Geometry: final body of the model. Coordinates: model frame, mm. Face numbers are marked on the shaded views. Round coordinates to 2 decimals unless told otherwise and drop trailing zeros. Write each loop counter-clockwise with the first axis right and the second up, starting at its lowest first coordinate (ties: lowest second). Pieces come first, ordered by that corner, then holes. Notation, with made-up numbers: M 46.25,57 L 71.25,57 A13 cw 71.25,67 Z; hole C -13,40.25 d10. An arc over 180 degrees is marked long. Use one line per item in the form item = value. Start each with the question number.
Item 1: Ray query, probe 1 along X at (y, z) = (3.8, 20); probe 2 along Z at (x, y) = (-13.5, -6.25); probe 3 along X at (y, z) = (-5.25, -16.5). Return the intervals inside material, ascending.
Item 2: Section query A-A (y = -10.5). Return loops of the section in (x, z).
Item 3: Section query D-D (y = -2.25). State how many separate pieces and enclosed holes the cut face has, and give its area (3 significant figures).
Item 4: Pin query (flat end, axial travel): pin 1 Ø5 at (y, z) = (-8, 22.5) entering from -X; pin 2 Ø1.3 at (x, z) = (-32.5, -20) entering from +Y; pin 3 Ø0.5 at (x, y) = (-37.5, -5.5) entering from -Z; pin 4 Ø4.5 at (x, z) = (-34.5, 20) entering from -Y. Return the tip coordinate at first contact, or that it passes through.
Item 5: Pull-direction query (Z, two-part tool) for the marked faces 1, 2, 3 and 4; classes: pulls with the +Z half, pulls with the -Z half, needs draft (parallel to the pull), parting line crosses it, or undercut.
Item 6: Section query C-C (x = -13.5). Return loops of the section in (y, z), and give its area (3 significant figures).
Item 7: Section query B-B (z = 1). Return loops of the section in (x, y), and give its area (3 significant figures).
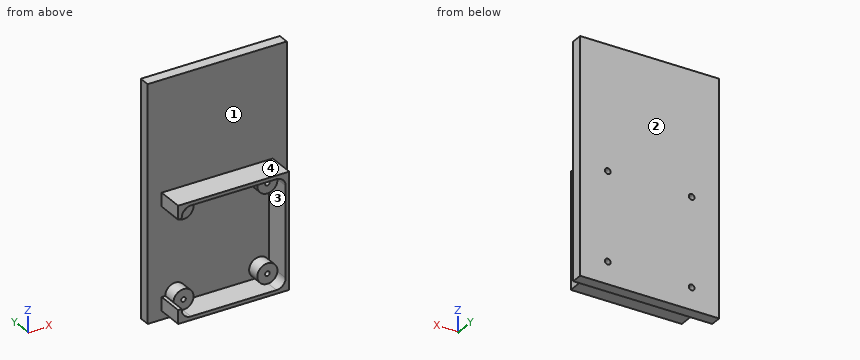
from build123d import *

# Parameters (mm, degrees)
SKETCH3_W           = 63
SKETCH3_H           = 60
BOSS_EXTRUDE3_DEPTH = 5
CUT_EXTRUDE1_REACH  = 56.314
SKETCH4_R           = 1.3
SKETCH9_R           = 4.55
SKETCH9_R_2         = 1.05
BOSS_EXTRUDE5_DEPTH = 6
SKETCH11_W          = 63
SKETCH11_H          = 5
BOSS_EXTRUDE7_DEPTH = 46
SKETCH12_W          = 50.3
SKETCH12_H          = 52.3
BOSS_EXTRUDE8_DEPTH = 12
SKETCH13_W          = 40
SKETCH13_H          = 12
CUT_EXTRUDE4_DEPTH  = 1.62


with BuildPart() as part:
    # Sketch3 → Boss-Extrude3 (new body)
    with BuildSketch(Plane(origin=(0, 0, 0), x_dir=(1, 0, 0), z_dir=(0, 1, 0))):
        with Locations((-13.5, 0)):
            Rectangle(SKETCH3_W, SKETCH3_H)
    extrude(amount=BOSS_EXTRUDE3_DEPTH)

    # Sketch4 → Cut-Extrude1 (cut, up to next)
    with BuildSketch(Plane(origin=(0, 5, 0), x_dir=(1, 0, 0), z_dir=(0, 1, 0)), mode=Mode.PRIVATE) as cut_extrude1_sk1:
        with Locations(Location((-32.5, 20, 0), (0, 0, 270))):
            Circle(SKETCH4_R)
    cut_extrude1_tool1 = extrude(cut_extrude1_sk1.sketch, amount=-CUT_EXTRUDE1_REACH, mode=Mode.PRIVATE) & part.part
    # Sketch4 → Cut-Extrude1 (cut, up to next)
    with BuildSketch(Plane(origin=(0, 5, 0), x_dir=(1, 0, 0), z_dir=(0, 1, 0)), mode=Mode.PRIVATE) as cut_extrude1_sk2:
        with Locations(Location((5.5, 20, 0), (0, 0, 270))):
            Circle(SKETCH4_R)
    cut_extrude1_tool2 = extrude(cut_extrude1_sk2.sketch, amount=-CUT_EXTRUDE1_REACH, mode=Mode.PRIVATE) & part.part
    # Sketch4 → Cut-Extrude1 (cut, up to next)
    with BuildSketch(Plane(origin=(0, 5, 0), x_dir=(1, 0, 0), z_dir=(0, 1, 0)), mode=Mode.PRIVATE) as cut_extrude1_sk3:
        with Locations(Location((5.5, -20, 0), (0, 0, 270))):
            Circle(SKETCH4_R)
    cut_extrude1_tool3 = extrude(cut_extrude1_sk3.sketch, amount=-CUT_EXTRUDE1_REACH, mode=Mode.PRIVATE) & part.part
    # Sketch4 → Cut-Extrude1 (cut, up to next)
    with BuildSketch(Plane(origin=(0, 5, 0), x_dir=(1, 0, 0), z_dir=(0, 1, 0)), mode=Mode.PRIVATE) as cut_extrude1_sk4:
        with Locations(Location((-32.5, -20, 0), (0, 0, 270))):
            Circle(SKETCH4_R)
    cut_extrude1_tool4 = extrude(cut_extrude1_sk4.sketch, amount=-CUT_EXTRUDE1_REACH, mode=Mode.PRIVATE) & part.part
    add(cut_extrude1_tool1.solids().sort_by_distance((-32.5, 5, -20))[0], mode=Mode.SUBTRACT)
    add(cut_extrude1_tool2.solids().sort_by_distance((5.5, 5, -20))[0], mode=Mode.SUBTRACT)
    add(cut_extrude1_tool3.solids().sort_by_distance((5.5, 5, 20))[0], mode=Mode.SUBTRACT)
    add(cut_extrude1_tool4.solids().sort_by_distance((-32.5, 5, 20))[0], mode=Mode.SUBTRACT)

    # Sketch9 → Boss-Extrude5 (add)
    # profile 1 of 4: a face of its own
    with BuildSketch(Plane.XZ):
        with Locations(Location((-32.5, 20, 0), (0, 0, 270))):
            Circle(SKETCH9_R)
        with Locations(Location((-32.5, 20, 0), (0, 0, 270))):
            Circle(SKETCH9_R_2, mode=Mode.SUBTRACT)
    # profile 2 of 4: a face of its own
    with BuildSketch(Plane.XZ):
        with Locations(Location((-32.5, -20, 0), (0, 0, 270))):
            Circle(SKETCH9_R)
        with Locations(Location((-32.5, -20, 0), (0, 0, 270))):
            Circle(SKETCH9_R_2, mode=Mode.SUBTRACT)
    # profile 3 of 4: a face of its own
    with BuildSketch(Plane.XZ):
        with Locations(Location((5.5, 20, 0), (0, 0, 270))):
            Circle(SKETCH9_R)
        with Locations(Location((5.5, 20, 0), (0, 0, 270))):
            Circle(SKETCH9_R_2, mode=Mode.SUBTRACT)
    # profile 4 of 4: a face of its own
    with BuildSketch(Plane.XZ):
        with Locations(Location((5.5, -20, 0), (0, 0, 270))):
            Circle(SKETCH9_R)
        with Locations(Location((5.5, -20, 0), (0, 0, 270))):
            Circle(SKETCH9_R_2, mode=Mode.SUBTRACT)
    extrude(amount=BOSS_EXTRUDE5_DEPTH)

    # Sketch11 → Boss-Extrude7 (add)
    with BuildSketch(Plane.XY.offset(30)):
        with Locations((-13.5, 2.5)):
            Rectangle(SKETCH11_W, SKETCH11_H)
    extrude(amount=BOSS_EXTRUDE7_DEPTH)

    # Sketch12 → Boss-Extrude8 (add)
    with BuildSketch(Plane.XZ):
        with Locations((-13.5, 0)):
            Rectangle(SKETCH12_W, SKETCH12_H)
        with BuildLine():
            Line((-32.889447937, 24.533302362), (5.889447937, 24.533302362))
            ThreePointArc((5.889447937, 24.533302362), (8.819595501, 23.319595501), (10.033302362, 20.389447937))
            Line((10.033302362, 20.389447937), (10.033302362, -20.389447937))
            ThreePointArc((10.033302362, -20.389447937), (8.819595501, -23.319595501), (5.889447937, -24.533302362))
            Line((5.889447937, -24.533302362), (-32.889447937, -24.533302362))
            ThreePointArc((-32.889447937, -24.533302362), (-35.819595501, -23.319595501), (-37.033302362, -20.389447937))
            Line((-37.033302362, -20.389447937), (-37.033302362, 20.389447937))
            ThreePointArc((-37.033302362, 20.389447937), (-35.819595501, 23.319595501), (-32.889447937, 24.533302362))
        make_face(mode=Mode.SUBTRACT)
    extrude(amount=BOSS_EXTRUDE8_DEPTH)

    # Sketch13 → Cut-Extrude4 (cut)
    with BuildSketch(Plane.ZY.offset(38.65)):
        with Locations((0, -6)):
            Rectangle(SKETCH13_W, SKETCH13_H)
    extrude(amount=-CUT_EXTRUDE4_DEPTH, mode=Mode.SUBTRACT)


solid = part.part
Working result:
q1.probe_1 = -45 to -33.8, -31.2 to 4.2, 6.8 to 18
q1.probe_2 = -26.15 to -24.53, 24.53 to 26.15
q1.probe_3 = -35.41 to -29.59, 2.59 to 8.41, 10.03 to 11.65
q2.outline = M -38.65,-26.15 L 11.65,-26.15 L 11.65,26.15 L -38.65,26.15 L -38.65,20 L -37.03,20 L -37.03,20.39 A4.14 cw -32.89,24.53 L 5.89,24.53 A4.14 cw 10.03,20.39 L 10.03,-20.39 A4.14 cw 5.89,-24.53 L -32.89,-24.53 A4.14 cw -37.03,-20.39 L -37.03,-20 L -38.65,-20 Z
q3.separate_pieces = 1
q3.enclosed_holes = 8
q3.area = 518 mm²
q4.pin_1 = -38.65
q4.pin_2 = through
q4.pin_3 = -26.15
q4.pin_4 = -6
q5.face_1 = undercut
q5.face_2 = needs draft
q5.face_3 = undercut
q5.face_4 = pulls with the +Z half
q6.outline = M -12,-26.15 L 0,-26.15 L 0,-30 L 5,-30 L 5,76 L 0,76 L 0,26.15 L -12,26.15 L -12,24.53 L 0,24.53 L 0,-24.53 L -12,-24.53 Z
q6.area = 569 mm²
q7.outline = M -45,0 L 10.03,0 L 10.03,-12 L 11.65,-12 L 11.65,0 L 18,0 L 18,5 L -45,5 Z
q7.area = 334 mm²
